```python
from build123d import *

# Parameters (mm, degrees)
PAD_DEPTH       = 9.88
SKETCH001_W     = 2.75
SKETCH001_H     = 2.75
POCKET_DEPTH    = 20
FILLET_R        = 1
CHAMFER_SIZE    = 0.5
CHAMFER001_SIZE = 0.25


with BuildPart() as foot:
    # Sketch → Pad (new body)
    with BuildSketch(Plane.YZ):
        Polygon((1.57769, 8.947526), (0.883098, 5.008295), (0, 0), (-1.575692, 0.277837), (-6.575692, 0.277837), (-6.575692, -4.722163), (28.424308, -4.722163), (28.424308, 4.213743), align=None)
    extrude(amount=PAD_DEPTH)

    # Sketch001 (on Face9 of Pad) → Pocket (cut)
    with BuildSketch(Plane(origin=(0, 0, 0), x_dir=(0, -0.173648, -0.984808), z_dir=(0, -0.984808, 0.173648))):
        with Locations((-5.087502, 4.946713)):
            Rectangle(SKETCH001_W, SKETCH001_H)
    extrude(amount=-POCKET_DEPTH, mode=Mode.SUBTRACT)

    # Fillet
    fillet_edges = [foot.edges().sort_by_distance(p)[0] for p in [
        (9.88, -4.075692, 0.277837),
        (4.94, -6.575692, 0.277837),
        (0, -4.075692, 0.277837),
        (4.94, 1.57769, 8.947526),
        (0, 15.000999, 6.580635),
        (9.88, 15.000999, 6.580635),
        (9.88, 0.788845, 4.473763),
        (0, 0.788845, 4.473763),
        (4.94, 28.424308, 4.213743),
        (9.88, 28.424308, -0.25421),
        (9.88, -0.787846, 0.138919),
        (0, -0.787846, 0.138919),
        (9.88, -6.575692, -2.222163),
        (0, -6.575692, -2.222163),
        (0, 28.424308, -0.25421),
    ]]
    fillet(fillet_edges, radius=FILLET_R)

    # Chamfer
    chamfer_edges = [foot.edges().sort_by_distance(p)[0] for p in [
        (0, 10.924308, -4.722163),
    ]]
    chamfer(chamfer_edges, length=CHAMFER_SIZE)

    # Chamfer001
    chamfer001_edges = [foot.edges().sort_by_distance(p)[0] for p in [
        (3.571713, 0.883435, 5.010211),
        (4.946713, 1.122202, 6.364322),
        (6.321713, 0.883435, 5.010211),
        (4.946713, 0.644669, 3.656101),
    ]]
    chamfer(chamfer001_edges, length=CHAMFER001_SIZE)


with BuildPart() as foot_1:
    # Body placement: moved
    add(foot.part.moved(Location((-34.3, 0, 0))))


with BuildPart() as foot_mirror:
    # Part__Mirroring: instance of Foot
    add(foot_1.part.mirror(Plane(origin=(0, 0, 0), x_dir=(0, -1, 0), z_dir=(1, 0, 0))))


solid = foot_mirror.part
```
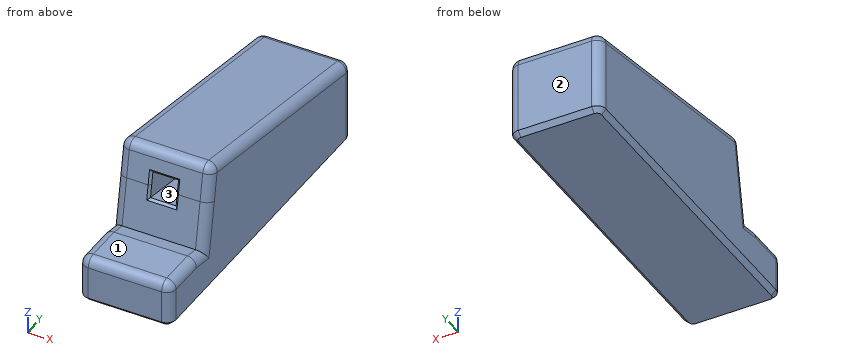
Model file for the job. Use its own axes, mm. Face numbers are marked on the shaded views. Coordinates: 2 decimals unless noted, no trailing zeros. Loops run counter-clockwise (first coordinate to the right, second up) from the corner with the lowest first, then second, coordinate; pieces in that order, holes last. Notation, with made-up numbers: (61.25, 69) - (66.25, 69) arc R28 ccw to (66.25, 99) - close; hole circle Ø4 at (-30.5, -14.5). An arc over 180 degrees is marked (long way). Write item = value, one per line. Start each with the question number.
Item 1: Pull direction Y, two halves, no side cores. Call the marked faces 1, 2 and 3: +Y half, -Y half, draft (parallel to the pull), parting line (faces both ways), or undercut.
Item 2: Saw through at B-B, the plane y = -3. List the corners of the cut face in (x, z), then the cut area to 3 significant figures.
Item 3: Saw through at C-C, the plane x = 28.5. List the corners of the cut face in (y, z), then the cut area to 3 significant figures.
Item 4: Saw through at A-A, the plane x = 26.25. List the corners of the cut face in (y, z).
Item 5: Wall check: probe 1 along X at (y, z) = (10.5, 2.25); probe 2 along Z at (x, y) = (30, 11); probe 3 along Z at (x, y) = (27.5, -1). Give the ranges that are in metal, low to high. Write a range as [from, to].
Item 6: Drop a flat-ended pin along its axis: pin 1 Ø3 at (x, y) = (31, -4) entering from +Z. Give the stop position or say it passes through.
Answers:
q1.face_1 = draft
q1.face_2 = +Y half
q1.face_3 = undercut
q2.outline = (24.42, -4.22) - (24.92, -4.72) - (33.8, -4.72) - (34.3, -4.22) - (34.3, -0.72) arc R1 ccw to (33.3, 0.28) - (25.42, 0.28) arc R1 ccw to (24.42, -0.72) - close
q2.area = 48.7 mm2
q3.outline = (-6.58, -4.22) - (-6.08, -4.72) - (27.92, -4.72) - (28.42, -4.22) - (28.42, 3.37) arc R1 ccw to (27.6, 4.36) - (2.56, 8.77) arc R1 ccw to (1.4, 7.96) - (1.17, 6.61) - (1.37, 6.32) - (20.82, 2.89) - (20.34, 0.18) - (0.89, 3.61) - (0.6, 3.41) - (0, 0) - (-1.58, 0.28) - (-5.58, 0.28) arc R1 ccw to (-6.58, -0.72) - close
q3.area = 295 mm2
q4.outline = (-6.58, -4.22) - (-6.08, -4.72) - (27.92, -4.72) - (28.42, -4.22) - (28.42, 3.37) arc R1 ccw to (27.6, 4.36) - (2.56, 8.77) arc R1 ccw to (1.4, 7.96) - (0.88, 5.01) - (0, 0) - (-1.58, 0.28) - (-5.58, 0.28) arc R1 ccw to (-6.58, -0.72) - close
q5.probe_1 = [24.42, 27.98], [30.73, 34.3]
q5.probe_2 = [-4.72, 1.83], [4.62, 7.29]
q5.probe_3 = [-4.72, 0.18]
q6.pin_1 = 0.28
